```python
from build123d import *

# Parameters (mm, degrees)
CROQUIS1_W                 = 416
CROQUIS1_H                 = 294
SALIENTE_EXTRUIR1_DEPTH    = 5
CORTAR_EXTRUIR1_DEPTH      = 255.750858684
REDONDEO1_R                = 10
SALIENTE_EXTRUIR3_DEPTH    = 20
REDONDEO2_R                = 5
REDONDEO2_OF_SIMETR_A3_R   = 5
CORTAR_EXTRUIR5_DEPTH      = 256.925770488
CORTAR_EXTRUIR5_DEPTH_BACK = 256.925770488
REDONDEO4_R                = 20
ESCALA1_START              = -20
ESCALA1_DEPTH              = 17.828103166
ESCALA1_START_2            = -2.171896834
ESCALA1_2_DEPTH            = 10
ESCALA1_START_3            = -42.171896834
ESCALA1_3_DEPTH            = 40
CROQUIS9_W                 = 50
CROQUIS9_H                 = 50
SALIENTE_EXTRUIR4_DEPTH    = 2
REDONDEO5_R                = 5
CROQUIS10_R                = 2
CORTAR_EXTRUIR7_DEPTH      = 2
CROQUIS11_R                = 20
SALIENTE_EXTRUIR5_DEPTH    = 3
CROQUIS12_R                = 16
CORTAR_EXTRUIR8_DEPTH      = 3
CROQUIS13_R                = 20
SALIENTE_EXTRUIR6_DEPTH    = 2
CROQUIS14_R                = 18
CORTAR_EXTRUIR9_DEPTH      = 2


# Read off the part's stored shape, not the designer's step: Escala1
with BuildPart() as part:
    # Croquis1 → Saliente-Extruir1 (new body)
    with BuildSketch(Plane(origin=(0, 0, 0), x_dir=(1, 0, 0), z_dir=(0, 1, 0))):
        Rectangle(CROQUIS1_W, CROQUIS1_H)
    extrude(amount=SALIENTE_EXTRUIR1_DEPTH)

    # Croquis3 → Cortar-Extruir1 (cut, through all)
    with BuildSketch(Plane(origin=(0, 5, 0), x_dir=(1, 0, 0), z_dir=(0, 1, 0))):
        with BuildLine():
            Line((-193, 154.47), (-193, 134.47))
            Line((-193, 134.47), (-148, 134.47))
            Line((-148, 134.47), (-148, 129.47))
            Line((-148, 129.47), (-133, 129.47))
            Line((-133, 129.47), (-133, 134.47))
            Line((-133, 134.47), (-118, 134.47))
            ThreePointArc((-118, 134.47), (-111.127739024, 134.944531511), (-104.385922224, 136.359118837))
            Line((-104.385922224, 136.359118837), (-104, 156.355395091))
            Line((-104, 156.355395091), (-193, 156.355395091))
            Line((-193, 156.355395091), (-193, 154.47))
        make_face()
    cortar_extruir1 = extrude(amount=-CORTAR_EXTRUIR1_DEPTH, mode=Mode.SUBTRACT)

    # Simetría1: Cortar-Extruir1 across plane
    add(cortar_extruir1.mirror(Plane.XY), mode=Mode.SUBTRACT)

    # Redondeo1
    redondeo1_edges = [part.edges().sort_by_distance(p)[0] for p in [
        (-208, 2.5, -147),
        (208, 2.5, -147),
        (208, 2.5, 147),
        (-208, 2.5, 147),
    ]]
    fillet(redondeo1_edges, radius=REDONDEO1_R)

    # Croquis5 → Saliente-Extruir3 (add)
    with BuildSketch(Plane.XZ):
        Polygon((-208, 110.96), (-115, 110.96), (-115, 134.560081146), (-118, 134.47), (-118, 113.96), (-208, 113.96), align=None)
    saliente_extruir3 = extrude(amount=SALIENTE_EXTRUIR3_DEPTH)

    # Redondeo2
    redondeo2_edges = [part.edges().sort_by_distance(p)[0] for p in [
        (-115, -10, 110.96),
    ]]
    fillet(redondeo2_edges, radius=REDONDEO2_R)

    # Simetría3: Saliente-Extruir3 across plane
    add(saliente_extruir3.mirror(Plane.XY))

    # Redondeo2 of Simetría3
    redondeo2_of_simetr_a3_edges = [part.edges().sort_by_distance(p)[0] for p in [
        (-115, -10, -110.96),
    ]]
    fillet(redondeo2_of_simetr_a3_edges, radius=REDONDEO2_OF_SIMETR_A3_R)

    # Croquis7 → Cortar-Extruir5 (cut, two sides: drawn at the far end of the back side and taken through both)
    with BuildSketch(Plane(origin=(0, 5, 0), x_dir=(1, 0, 0), z_dir=(0, 1, 0)).offset(-CORTAR_EXTRUIR5_DEPTH_BACK)):
        with BuildLine():
            Line((198, 147), (0, 147))
            add(Edge.make_bspline(
                [(0, 147), (208, 73.5), (208, 0)],
                knots=[0, 0, 0, 0.5, 0.5, 0.5], degree=2))
            Line((208, 0), (208, 137))
            ThreePointArc((208, 137), (205.071067812, 144.071067812), (198, 147))
        make_face()
        with BuildLine():
            Line((208, -137), (208, 0))
            add(Edge.make_bspline(
                [(208, 0), (208, -73.5), (0, -147)],
                knots=[0.5, 0.5, 0.5, 1, 1, 1], degree=2))
            Line((0, -147), (198, -147))
            ThreePointArc((198, -147), (205.071067812, -144.071067812), (208, -137))
        make_face()
    extrude(amount=CORTAR_EXTRUIR5_DEPTH + CORTAR_EXTRUIR5_DEPTH_BACK, mode=Mode.SUBTRACT)

    # Redondeo4
    redondeo4_edges = [part.edges().sort_by_distance(p)[0] for p in [
        (0, 2.5, -147),
        (0, 2.5, 147),
    ]]
    fillet(redondeo4_edges, radius=REDONDEO4_R)

    # Escala1 outline → Escala1 (cut)
    with BuildSketch(Plane(origin=(0, 0, 0), x_dir=(1, 0, 0), z_dir=(0, 1, 0)).offset(ESCALA1_START)):
        with BuildLine():
            Line((-115, 115.96), (-115, 134.560081146))
            Line((-115, 134.560081146), (-118, 134.47))
            Line((-118, 134.47), (-118, 113.96))
            Line((-118, 113.96), (-208, 113.96))
            Line((-208, 113.96), (-208, 110.96))
            Line((-208, 110.96), (-120, 110.96))
            ThreePointArc((-120, 110.96), (-116.464466094, 112.424466094), (-115, 115.96))
        make_face()
        with BuildLine():
            Line((-118, -134.47), (-115, -134.560081146))
            Line((-115, -134.560081146), (-115, -115.96))
            ThreePointArc((-115, -115.96), (-116.464466094, -112.424466094), (-120, -110.96))
            Line((-120, -110.96), (-208, -110.96))
            Line((-208, -110.96), (-208, -113.96))
            Line((-208, -113.96), (-118, -113.96))
            Line((-118, -113.96), (-118, -134.47))
        make_face()
    extrude(amount=ESCALA1_DEPTH, mode=Mode.SUBTRACT)

    # Escala1 2 outline → Escala1 2 (add)
    with BuildSketch(Plane(origin=(0, 0, 0), x_dir=(1, 0, 0), z_dir=(0, 1, 0)).offset(ESCALA1_START_2)):
        with BuildLine():
            add(Edge.make_bspline(
                [(36.105170669, 291.681097591), (855.032944113, -0.000122107), (36.105170669, -291.681341805)],
                knots=[0.003943504, 0.003943504, 0.003943504, 0.996056496, 0.996056496, 0.996056496], degree=2))
            ThreePointArc((36.105170669, 291.681097591), (29.49404346, 293.415920236), (22.684079728, 293.999877893))
            Line((22.684079728, 293.999877893), (-178.792055331, 293.999877893))
            Line((-178.792055331, 293.999877893), (-179.202787056, 272.718115567))
            ThreePointArc((-179.202787056, 272.718115567), (-192.686420657, 269.888940914), (-206.430942609, 268.939877893))
            Line((-206.430942609, 268.939877893), (-236.430942609, 268.939877893))
            Line((-236.430942609, 268.939877893), (-236.430942609, 258.939877893))
            Line((-236.430942609, 258.939877893), (-266.430942609, 258.939877893))
            Line((-266.430942609, 258.939877893), (-266.430942609, 268.939877893))
            Line((-266.430942609, 268.939877893), (-356.430942609, 268.939877893))
            Line((-356.430942609, 268.939877893), (-356.430942609, 293.999877893))
            Line((-356.430942609, 293.999877893), (-366.430942609, 293.999877893))
            ThreePointArc((-366.430942609, 293.999877893), (-380.573078233, 288.142013517), (-386.430942609, 273.999877893))
            Line((-386.430942609, 273.999877893), (-386.430942609, -274.000122107))
            ThreePointArc((-386.430942609, -274.000122107), (-380.573078233, -288.142257731), (-366.430942609, -294.000122107))
            Line((-366.430942609, -294.000122107), (-356.430942609, -294.000122107))
            Line((-356.430942609, -294.000122107), (-356.430942609, -268.940122107))
            Line((-356.430942609, -268.940122107), (-266.430942609, -268.940122107))
            Line((-266.430942609, -268.940122107), (-266.430942609, -258.940122107))
            Line((-266.430942609, -258.940122107), (-236.430942609, -258.940122107))
            Line((-236.430942609, -258.940122107), (-236.430942609, -268.940122107))
            Line((-236.430942609, -268.940122107), (-206.430942609, -268.940122107))
            ThreePointArc((-206.430942609, -268.940122107), (-192.686420657, -269.889185129), (-179.202787056, -272.718359781))
            Line((-179.202787056, -272.718359781), (-178.792055331, -294.000122107))
            Line((-178.792055331, -294.000122107), (22.684079728, -294.000122107))
            ThreePointArc((22.684079728, -294.000122107), (29.49404346, -293.41616445), (36.105170669, -291.681341805))
        make_face()
    extrude(amount=ESCALA1_2_DEPTH)

    # Escala1 3 outline → Escala1 3 (add)
    with BuildSketch(Plane(origin=(0, 0, 0), x_dir=(1, 0, 0), z_dir=(0, 1, 0)).offset(ESCALA1_START_3)):
        with BuildLine():
            Line((-200.430942609, 231.919877893), (-200.430942609, 269.120040185))
            Line((-200.430942609, 269.120040185), (-206.430942609, 268.939877893))
            Line((-206.430942609, 268.939877893), (-206.430942609, 227.919877893))
            Line((-206.430942609, 227.919877893), (-386.430942609, 227.919877893))
            Line((-386.430942609, 227.919877893), (-386.430942609, 221.919877893))
            Line((-386.430942609, 221.919877893), (-210.430942609, 221.919877893))
            ThreePointArc((-210.430942609, 221.919877893), (-203.359874797, 224.848810081), (-200.430942609, 231.919877893))
        make_face()
        with BuildLine():
            Line((-206.430942609, -268.940122107), (-200.430942609, -269.120284399))
            Line((-200.430942609, -269.120284399), (-200.430942609, -231.920122107))
            ThreePointArc((-200.430942609, -231.920122107), (-203.359874797, -224.849054295), (-210.430942609, -221.920122107))
            Line((-210.430942609, -221.920122107), (-386.430942609, -221.920122107))
            Line((-386.430942609, -221.920122107), (-386.430942609, -227.920122107))
            Line((-386.430942609, -227.920122107), (-206.430942609, -227.920122107))
            Line((-206.430942609, -227.920122107), (-206.430942609, -268.940122107))
        make_face()
    extrude(amount=ESCALA1_3_DEPTH)

    # Croquis9 → Saliente-Extruir4 (add)
    with BuildSketch(Plane.XZ.offset(2.171896834)):
        with Locations((250, 0)):
            Rectangle(CROQUIS9_W, CROQUIS9_H)
    extrude(amount=SALIENTE_EXTRUIR4_DEPTH)

    # Redondeo5
    redondeo5_edges = [part.edges().sort_by_distance(p)[0] for p in [
        (275, -3.171896834, -25),
        (275, -3.171896834, 25),
        (225, -3.171896834, 25),
        (225, -3.171896834, -25),
    ]]
    fillet(redondeo5_edges, radius=REDONDEO5_R)

    # Croquis10 → Cortar-Extruir7 (cut)
    with BuildSketch(Plane.XZ.offset(4.171896834)):
        with Locations(Location((230, 20, 0), (0, 0, 270))):
            Circle(CROQUIS10_R)
        with Locations(Location((270, 20, 0), (0, 0, 270))):
            Circle(CROQUIS10_R)
    cortar_extruir7 = extrude(amount=-CORTAR_EXTRUIR7_DEPTH, mode=Mode.SUBTRACT)

    # Simetría7: Cortar-Extruir7 across plane
    add(cortar_extruir7.mirror(Plane.XY), mode=Mode.SUBTRACT)

    # Croquis11 → Saliente-Extruir5 (add)
    with BuildSketch(Plane.XZ.offset(4.171896834)):
        with Locations(Location((250, 0, 0), (0, 0, 270))):
            Circle(CROQUIS11_R)
    extrude(amount=SALIENTE_EXTRUIR5_DEPTH)

    # Croquis12 → Cortar-Extruir8 (cut)
    with BuildSketch(Plane.XZ.offset(7.171896834)):
        with Locations(Location((250, 0, 0), (0, 0, 270))):
            Circle(CROQUIS12_R)
    extrude(amount=-CORTAR_EXTRUIR8_DEPTH, mode=Mode.SUBTRACT)

    # Croquis13 → Saliente-Extruir6 (add)
    with BuildSketch(Plane.XZ.offset(4.171896834)):
        with Locations(Location((250, 0, 0), (0, 0, 270))):
            Circle(CROQUIS13_R)
    extrude(amount=SALIENTE_EXTRUIR6_DEPTH)

    # Croquis14 → Cortar-Extruir9 (cut)
    with BuildSketch(Plane.XZ.offset(6.171896834)):
        with Locations(Location((250, 0, 0), (0, 0, 270))):
            Circle(CROQUIS14_R)
    extrude(amount=-CORTAR_EXTRUIR9_DEPTH, mode=Mode.SUBTRACT)


solid = part.part
```
Geometry check sheet. Reference: the model listing, model coordinates, mm. A direction names the side the tool comes from. Give positions to 0.01 mm unless a question says otherwise; leave off trailing zeros. Order: outer loops, then holes, each group sorted by start corner. A loop starts at its lowest first (then second) coordinate and runs counter-clockwise, first axis right, second up. Notation, with made-up numbers: (69.25, -21.5) - (119.25, -21.5) arc R5 ccw to (119.25, -15.5) - close; hole circle Ø2 at (80, 53.25). An arc over 180 degrees is marked (long way). Answer in a Markdown table with one row per item. Add a question column.
Q1. Gauge pin test, flat ends, axial feed: pin 1 (8 mm diameter, centred on x = -315, y = 4.5, fed in from +Z); pin 2 (3 mm diameter, centred on x = 208, z = -157, fed in from -Y); pin 3 (12 mm diameter, centred on y = -24, z = -249, fed in from -X). Record the tip position at first contact, or that the pin passes through.
Q2. Cross-section at C-C, the plane x = -62.5. Enter the section's corners in (y, z), then the cut area to 3 significant figures.
Q3. Material ranges on probe 1 along X at (y, z) = (-3.55, -20); probe 2 along Z at (x, y) = (270, -3); probe 3 along X at (y, z) = (-5.15, 0), recorded low to high. Write a range as from..to.
Q4. Cross-section at B-B, the plane x = -292. Enter the section's corners in (y, z), then the cut area to 3 significant figures.
Q5. Cross-section at A-A, the plane y = -18. Enter the section's corners in (x, z), then the cut area to 3 significant figures.
Q6. Mould release check, pull along X, two halves, no side actions. Record for faces 5 (the flat face through (-200.431, -22, -250)), 6 (the flat face through (239, -6.172, 12)), 7 (the flat face through (-33, 7.828, -4)), 8 (the cylindrical face through (267.847, -5.186, 2.343)): pulls with the +X half, pulls with the -X half, needs draft (parallel to the pull), parting line crosses it, or undercut.
Q7. Tool access check on faces 1 (the flat face through (-300, -22, -221.92)), 2 (the flat face through (-298, -22, 227.92)), 3 (the flat face through (250, -4.172, 0)), 4 (the cylindrical face through (234.38, -6.68, 3.47)). Record the directions out of +Z, -Z, +X, -X, +Y, -Y that give a thin tool (end or side, any length) a straight path to the whole face; none if there is none.
Check values:
| question | item | result |
|---|---|---|
| 1 | pin 1 | stops at z = 268.94 |
| 1 | pin 2 | stops at y = -2.17 |
| 1 | pin 3 | stops at x = -206.43 |
| 2 | outline | (-2.17, -294) - (7.83, -294) - (7.83, 294) - (-2.17, 294) - close |
| 2 | area | 5,880 mm^2 |
| 3 | probe 1 | x = 225..228, 232..268, 272..275 |
| 3 | probe 2 | z = -25..-22, -18..18, 22..25 |
| 3 | probe 3 | x = 230..232, 268..270 |
| 4 | outline | (-42.17, -227.92) - (-2.17, -227.92) - (-2.17, -268.94) - (7.83, -268.94) - (7.83, 268.94) - (-2.17, 268.94) - (-2.17, 227.92) - (-42.17, 227.92) - (-42.17, 221.92) - (-2.17, 221.92) - (-2.17, -221.92) - (-42.17, -221.92) - close |
| 4 | area | 5,860 mm^2 |
| 5 | outline | (-386.43, -227.92) - (-206.43, -227.92) - (-206.43, -268.94) - (-200.43, -269.12) - (-200.43, -231.92) arc R10 ccw to (-210.43, -221.92) - (-386.43, -221.92) - close; (-386.43, 221.92) - (-210.43, 221.92) arc R10 ccw to (-200.43, 231.92) - (-200.43, 269.12) - (-206.43, 268.94) - (-206.43, 227.92) - (-386.43, 227.92) - close |
| 5 | area | 2,680 mm^2 |
| 6 | face 5 | pulls with the +X half |
| 6 | face 6 | undercut |
| 6 | face 7 | needs draft |
| 6 | face 8 | undercut |
| 7 | face 1 | +X, -X, -Y |
| 7 | face 2 | +Z, -X, -Y |
| 7 | face 3 | none |
| 7 | face 4 | -Y |
